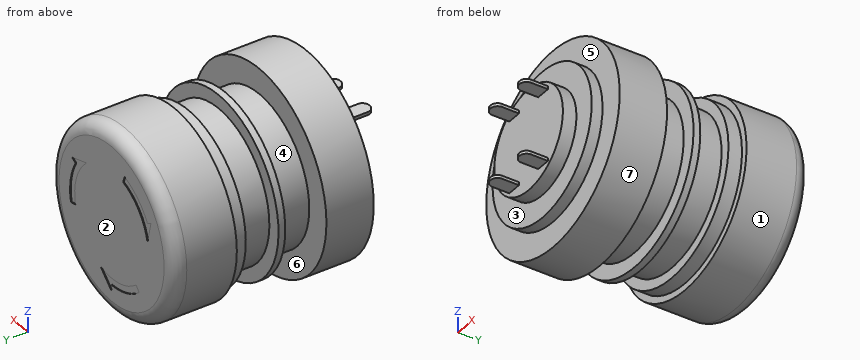
from build123d import *

# Parameters (mm, degrees)
SKETCH_1_R          = 7.5
EXTRUDE_1_DEPTH     = 2
SKETCH_2_W          = 2.124250946
SKETCH_2_H          = 0.455196631
EXTRUDE_2_DEPTH     = 3.5
FILLET_1_R          = 1
SKETCH_4_R          = 10.85
EXTRUDE_3_DEPTH     = 8.6
SKETCH_5_R          = 13
EXTRUDE_4_DEPTH     = 6
SKETCH_7_R          = 11
EXTRUDE_6_DEPTH     = 4.5
SKETCH_8_R          = 13.5
EXTRUDE_7_DEPTH     = 11.4
FILLET_5_R          = 2
SKETCH_9_OUTSIDE_W  = 39.496
SKETCH_9_OUTSIDE_H  = 39.496
SKETCH_9_OUTSIDE_R  = 12.5
CUT_EXTRUDE_1_DEPTH = 2
CUT_EXTRUDE_2_DEPTH = 0.1
SKETCH_11_R         = 14.605
EXTRUDE_8_DEPTH     = 7
SKETCH_12_R         = 13
SKETCH_12_R_2       = 10.85
CUT_EXTRUDE_3_DEPTH = 5


with BuildPart() as part:
    # 草图1 → 凸台-拉伸1 (new body)
    with BuildSketch(Plane(origin=(0, 0, 0), x_dir=(1, 0, 0), z_dir=(0, 1, 0))):
        with Locations(Location((0, 0, 0), (0, 0, 270))):
            Circle(SKETCH_1_R)
    extrude(amount=EXTRUDE_1_DEPTH)

    # 草图2 → 凸台-拉伸2 (add)
    with BuildSketch(Plane.XZ):
        with Locations((-3.169695017, 5.334335524)):
            Rectangle(SKETCH_2_W, SKETCH_2_H)
        with Locations((3.169695017, 5.334335524)):
            Rectangle(SKETCH_2_W, SKETCH_2_H)
        with Locations((3.169695017, -5.334335524)):
            Rectangle(SKETCH_2_W, SKETCH_2_H)
        with Locations((-3.169695017, -5.334335524)):
            Rectangle(SKETCH_2_W, SKETCH_2_H)
    extrude(amount=EXTRUDE_2_DEPTH)

    # 圆角1
    fillet_1_edges = [part.edges().sort_by_distance(p)[0] for p in [
        (4.23182049, -3.5, 5.334335524),
        (2.107569544, -3.5, 5.334335524),
        (4.23182049, -3.5, -5.334335524),
        (2.107569544, -3.5, -5.334335524),
        (-4.23182049, -3.5, -5.334335524),
        (-2.107569544, -3.5, -5.334335524),
        (-2.107569544, -3.5, 5.334335524),
        (-4.23182049, -3.5, 5.334335524),
    ]]
    fillet(fillet_1_edges, radius=FILLET_1_R)

    # 草图4 → 凸台-拉伸3 (add)
    with BuildSketch(Plane(origin=(0, 2, 0), x_dir=(1, 0, 0), z_dir=(0, 1, 0))):
        with Locations(Location((0, 0, 0), (0, 0, 90))):
            Circle(SKETCH_4_R)
    extrude(amount=EXTRUDE_3_DEPTH)

    # 草图5 → 凸台-拉伸4 (add)
    with BuildSketch(Plane(origin=(0, 10.6, 0), x_dir=(1, 0, 0), z_dir=(0, 1, 0))):
        with Locations(Location((0, 0, 0), (0, 0, 270))):
            Circle(SKETCH_5_R)
    extrude(amount=EXTRUDE_4_DEPTH)

    # 草图7 → 凸台-拉伸6 (add)
    with BuildSketch(Plane(origin=(0, 16.6, 0), x_dir=(1, 0, 0), z_dir=(0, 1, 0))):
        with Locations(Location((0, 0, 0), (0, 0, 270))):
            Circle(SKETCH_7_R)
    extrude(amount=EXTRUDE_6_DEPTH)

    # 草图8 → 凸台-拉伸7 (add)
    with BuildSketch(Plane(origin=(0, 21.1, 0), x_dir=(1, 0, 0), z_dir=(0, 1, 0))):
        with Locations(Location((0, 0, 0), (0, 0, 270))):
            Circle(SKETCH_8_R)
    extrude(amount=EXTRUDE_7_DEPTH)

    # 圆角5
    fillet_5_edges = [part.edges().sort_by_distance(p)[0] for p in [
        (0, 32.5, -13.5),
    ]]
    fillet(fillet_5_edges, radius=FILLET_5_R)

    # 草图9 outside → 切除-拉伸1 (cut)
    with BuildSketch(Plane.XZ.offset(-21.1)):
        Rectangle(SKETCH_9_OUTSIDE_W, SKETCH_9_OUTSIDE_H)
        with Locations(Location((0, 0, 0), (0, 0, 270))):
            Circle(SKETCH_9_OUTSIDE_R, mode=Mode.SUBTRACT)
    extrude(amount=-CUT_EXTRUDE_1_DEPTH, mode=Mode.SUBTRACT)

    # 草图10 → 切除-拉伸2 (cut)
    with BuildSketch(Plane(origin=(0, 32.5, 0), x_dir=(1, 0, 0), z_dir=(0, 1, 0))):
        with BuildLine():
            Line((0, 9.073721602), (0, 9.961907626))
            Line((0, 9.961907626), (2.376046015, 7.716176893))
            ThreePointArc((2.376046015, 7.716176893), (-1.712152333, 7.890089663), (-5.36056205, 6.037330123))
            Line((-5.36056205, 6.037330123), (-6.024513857, 6.785105489))
            ThreePointArc((-6.024513857, 6.785105489), (-3.222286879, 8.48229279), (0, 9.073721602))
        make_face()
        with BuildLine():
            Line((8.627265074, -4.980953813), (5.494382202, -5.915804656))
            ThreePointArc((5.494382202, -5.915804656), (7.689094253, -2.462277416), (7.908762283, 1.623717852))
            Line((7.908762283, 1.623717852), (8.888330649, 1.824829301))
            ThreePointArc((8.888330649, 1.824829301), (8.957024478, -1.450564099), (7.858073414, -4.536860801))
            Line((7.858073414, -4.536860801), (8.627265074, -4.980953813))
        make_face()
        with BuildLine():
            Line((-8.627265074, -4.980953813), (-7.870428217, -1.800372237))
            ThreePointArc((-7.870428217, -1.800372237), (-5.97694192, -5.427812247), (-2.548200233, -7.661047975))
            Line((-2.548200233, -7.661047975), (-2.863816792, -8.60993479))
            ThreePointArc((-2.863816792, -8.60993479), (-5.734737599, -7.031728691), (-7.858073414, -4.536860801))
            Line((-7.858073414, -4.536860801), (-8.627265074, -4.980953813))
        make_face()
    extrude(amount=-CUT_EXTRUDE_2_DEPTH, mode=Mode.SUBTRACT)

    # 草图11 → 凸台-拉伸8 (add)
    with BuildSketch(Plane.XZ.offset(-10.6)):
        with Locations(Location((0, 0, 0), (0, 0, 270))):
            Circle(SKETCH_11_R)
    extrude(amount=EXTRUDE_8_DEPTH)

    # 草图12 → 切除-拉伸3 (cut)
    with BuildSketch(Plane(origin=(0, 10.6, 0), x_dir=(1, 0, 0), z_dir=(0, 1, 0))):
        with Locations(Location((0, 0, 0), (0, 0, 270))):
            Circle(SKETCH_12_R)
        with Locations(Location((0, 0, 0), (0, 0, 270))):
            Circle(SKETCH_12_R_2, mode=Mode.SUBTRACT)
    extrude(amount=CUT_EXTRUDE_3_DEPTH, mode=Mode.SUBTRACT)


solid = part.part
Design review of the part built by this model. Coordinates are the model's own, in mm. Face numbers are marked on the shaded views. A direction names the side the tool comes from. Round coordinates to 2 decimals unless told otherwise and drop trailing zeros. Write each loop counter-clockwise with the first axis right and the second up, starting at its lowest first coordinate (ties: lowest second). Pieces come first, ordered by that corner, then holes. Notation, with made-up numbers: M 66.25,73.25 L 99.25,73.25 A24 ccw 99.25,84.25 Z; hole C 24,33 d10. An arc over 180 degrees is marked long. One line per item, written item: value. Start each with the question number.
1. Take a section at A-A on y = 18. State the section outline as (x, z) points.
2. Clearance check with flat-ended pins moving along their axes: P1, Ø12, axis at x = 2.5, z = -2.5, coming from the -Y side; P2, Ø1.1, axis at x = -3.5, y = -1, coming from the -Z side; P3, Ø8, axis at y = 23, z = 5.5, coming from the +X side; P4, Ø1.1, axis at x = -3.5, y = -1.5, coming from the +Z side. State where each tip first meets the part, or that it passes through.
3. Draft analysis for pull direction Y (two halves, no side actions). For the marked faces 5, 6 and 7, state which applies: pulls with the +Y half, pulls with the -Y half, needs draft (parallel to the pull), parting line crosses it, or undercut.
4. To check wall thickness, follow probe 1 along Y at (x, z) = (9, 7.25); probe 2 along X at (y, z) = (18, -1.75); probe 3 along Z at (x, y) = (0.25, 24.5). State the ranges of each line that lie inside material, in increasing order. Write a range as from..to.
5. For the marked faces 1, 2, 3 and 4, list the 3-axis set-ups (+Z, -Z, +X, -X, +Y, -Y) from which the entire face can be reached by the end or side of a thin tool; tool diameter is ignored.
6. Take a section at B-B on y = 14. State the section outline as (x, z) points.
Computed:
1. outline: C 0,0 d22
2. P1: stops at y = -3.5
2. P2: stops at z = -5.56
2. P3: stops at x = 13.42
2. P4: stops at z = 5.56
3. face 5: pulls with the -Y half
3. face 6: undercut
3. face 7: needs draft
4. probe 1: y = 3.6..10.6, 15.6..16.6, 21.1..32.5
4. probe 2: x = -10.86..10.86
4. probe 3: z = -13.5..13.5
5. face 1: +Y
5. face 2: +Z, -Z, +X, -X, +Y
5. face 3: -Y
5. face 4: none
6. outline: C 0,0 d21.7
